```python
from build123d import *

# Parameters (mm, degrees)
SKETCH1_W                    = 38.1
SKETCH1_H                    = 12.7
BOSS_EXTRUDE1_DEPTH          = 1.524
SKETCH2_R                    = 1.5875
CUT_EXTRUDE1_DEPTH           = 21.138211837
CHAMFER1_SIZE                = 1.27
F_10_0_1935_DIAMETER_HOLE1_D = 4.9149


# Read off the part's stored shape, not the designer's step: deleteface
with BuildPart() as part:
    # Sketch1 → Boss-Extrude1 (new body)
    with BuildSketch(Plane.XY):
        Rectangle(SKETCH1_W, SKETCH1_H)
    extrude(amount=-BOSS_EXTRUDE1_DEPTH)

    # Sketch2 → Cut-Extrude1 (cut, through all)
    with BuildSketch(Plane.XY):
        with Locations((-12.7, 0)):
            Circle(SKETCH2_R)
        with Locations((-4.233333333, 0)):
            Circle(SKETCH2_R)
        with Locations((4.233333333, 0)):
            Circle(SKETCH2_R)
        with Locations((12.7, 0)):
            Circle(SKETCH2_R)
    extrude(amount=-CUT_EXTRUDE1_DEPTH, mode=Mode.SUBTRACT)

    # Chamfer1
    chamfer1_edges = [part.edges().sort_by_distance(p)[0] for p in [
        (-14.2875, 0, 0),
        (-5.820833333, 0, 0),
        (2.645833333, 0, 0),
        (11.1125, 0, 0),
    ]]
    chamfer(chamfer1_edges, length=CHAMFER1_SIZE)

    # deleteface outline → deleteface (revolve)
    with BuildSketch(Plane(origin=(-4.233333333, 0, 0), x_dir=(1, 0, 0), z_dir=(0, -1, 0))):
        Polygon((0, -1.524), (1.5875, -1.524), (1.5875, -1.27), (2.8575, 0), (0, 0), align=None)
    revolve(axis=Axis((-4.233333333, 0, 0), (0, 0, 1)))

    # deleteface 2 outline → deleteface 2 (revolve)
    with BuildSketch(Plane(origin=(4.233333333, 0, 0), x_dir=(1, 0, 0), z_dir=(0, -1, 0))):
        Polygon((0, -1.524), (1.5875, -1.524), (1.5875, -1.27), (2.8575, 0), (0, 0), align=None)
    revolve(axis=Axis((4.233333333, 0, 0), (0, 0, 1)))

    # #10 (0.1935) Diameter Hole1 (through all)
    with Locations(Plane.XY):
        with Locations((-12.7, 0)):
            Hole(F_10_0_1935_DIAMETER_HOLE1_D / 2)


solid = part.part
```
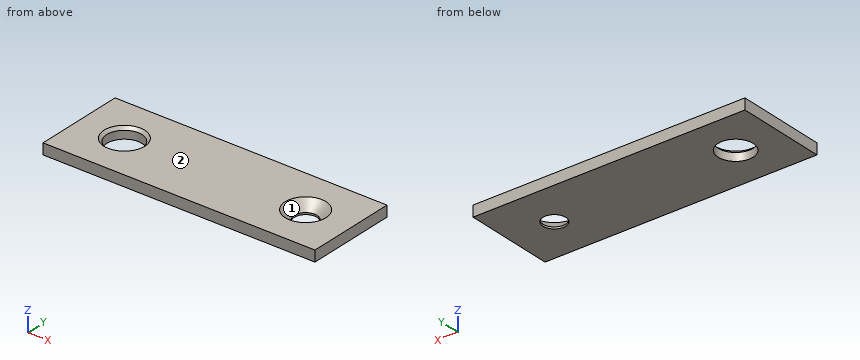
The model under review builds one solid part; all positions refer to its coordinate system, in mm. Face numbers are marked on the shaded views. Round coordinates to 2 decimals unless told otherwise and drop trailing zeros. Loops run counter-clockwise (first coordinate to the right, second up) from the corner with the lowest first, then second, coordinate; pieces in that order, holes last.
1) Consider section D-D on x = 12.7. State the section outline as (y, z) points, then the cut area to 3 significant figures.
Values follow:
outline: (-6.35, -1.52) - (-1.59, -1.52) - (-1.59, -1.27) - (-2.86, 0) - (-6.35, 0) - close; (1.59, -1.52) - (6.35, -1.52) - (6.35, 0) - (2.86, 0) - (1.59, -1.27) - close
area: 12.9 mm2
2) The part is to be moulded in two halves that separate along Y. For the marked faces 1 and 2, say which applies: pulls with the +Y half, pulls with the -Y half, needs draft (parallel to the pull), parting line crosses it, or undercut.
Values follow:
face 1: undercut
face 2: needs draft
3) Consider section A-A on y = 0. State the section outline as (x, z) points.
Values follow:
outline: (-19.05, -1.52) - (-15.16, -1.52) - (-15.16, -0.4) - (-15.56, 0) - (-19.05, 0) - close; (-10.24, -1.52) - (11.11, -1.52) - (11.11, -1.27) - (9.84, 0) - (-9.84, 0) - (-10.24, -0.4) - close; (14.29, -1.52) - (19.05, -1.52) - (19.05, 0) - (15.56, 0) - (14.29, -1.27) - close
4) Consider section B-B on x = -12.7. State the section outline as (y, z) points.
Values follow:
outline: (-6.35, -1.52) - (-2.46, -1.52) - (-2.46, -0.4) - (-2.86, 0) - (-6.35, 0) - close; (2.46, -1.52) - (6.35, -1.52) - (6.35, 0) - (2.86, 0) - (2.46, -0.4) - close
5) Consider section C-C on z = -0.7. Give the number of separate pieces and of enclosed holes in the cut face, then the cut area to 3 significant figures.
Values follow:
separate pieces: 1
enclosed holes: 2
area: 450 mm2
6) Wall thickness on line 1 along X through (y, z) = (0.25, -0.4); line 2 along Y through (x, z) = (-12.7, -1.05); line 3 along X through (y, z) = (0, -0.75): over which ranges is each line inside the solid? List them lowest first.
Values follow:
line 1: x = -19.05 to -15.14, -10.26 to 10.26, 15.14 to 19.05
line 2: y = -6.35 to -2.46, 2.46 to 6.35
line 3: x = -19.05 to -15.16, -10.24 to 10.59, 14.81 to 19.05
